Geometry: final body of the model. Coordinates: model frame, mm. A direction names the side the tool comes from. Give positions to 0.01 mm unless a question says otherwise; leave off trailing zeros. Write each loop counter-clockwise with the first axis right and the second up, starting at its lowest first coordinate (ties: lowest second). Pieces come first, ordered by that corner, then holes.
Autodesk Inventor part; units mm, degrees
ref_plane "YZ Plane" through (0, 0, 0) normal (1, 0, 0) x (0, 1, 0)
ref_plane "XZ Plane" through (0, 0, 0) normal (0, 1, 0) x (-1, 0, 0)
ref_plane "XY Plane" through (0, 0, 0) normal (0, 0, 1) x (1, 0, 0)
sketch "Skizze1" plane through (0, 0, 0) normal (0, 0, 1) x (1, 0, 0)
  line L0 (-17.5, 0) -> (17.5, 0)
  line L1 (0, -17.5) -> (0, 17.5)
  circle A0 centre (0, 0) radius 12.5
  dimension "d0" = 25
extrude "Extrusion1" add sketch "Skizze1" along normal blind 3
sketch "Skizze2" plane through (0, 0, 3) normal (0, 0, 1) x (1, 0, 0)
  circle A0 centre (0, 0) radius 10
  dimension "d3" = 20
extrude "Extrusion2" add sketch "Skizze2" along normal blind 5
thread "Gewinde1"
chamfer "Fase1" distance 0.5 angle 45 3 edges at (-10, 0, 8) (-12.5, 0, 3) (-12.5, 0, 0)
sketch "Skizze3" plane through (0, 0, 0) normal (0, 0, -1) x (-1, 0, 0)
  point P0 (0, 0)
  point P1 (0, 0)
hole "Bohrung1" at (0, 0, 0) direction (0, 0, 1) diameter 11.445 depth 32.814
properties part number "VerteilerVerschluss"
Q1. Pin query (flat end, axial travel): P1, Ø9, axis at x = 0, y = 0, coming from the -Z side; P2, Ø7, axis at x = -5.5, y = 0.5, coming from the +Z side; P3, Ø1, axis at y = 6.5, z = 1, coming from the +X side; P4, Ø1, axis at x = -9.5, z = 4, coming from the +Y side. Return the tip coordinate at first contact, or that it passes through.
Filled sheet:
P1: passes through
P2: stops at z = 8
P3: stops at x = 10.97
P4: stops at y = 4.36
Q2. Ray query, line 1 along Y through (x, z) = (0, 4); line 2 along Z through (x, y) = (-9.75, -5.75); line 3 along Y through (x, z) = (-3, 3.5). Return the intervals inside material, ascending.
Filled sheet:
line 1: y = -10 to -5.72, 5.72 to 10
line 2: z = 0 to 3
line 3: y = -9.54 to -4.87, 4.87 to 9.54
Q3. Access query for faces 4 (the flat face through (5.2, 2.8, 0)), 5 (the flat face through (-5, 9, 3)). Directions: +Z, -Z, +X, -X, +Y, -Y. A direction counts if a zero-diameter tool reaches every point of the face in a straight line with its end or side. Return the directions, or none.
Filled sheet:
face 4: -Z, +X, -X, +Y, -Y
face 5: +Z
Q4. Pull-direction query (X, two-part tool) for faces 1 (the flat face through (0, -6, 8)), 2 (the cylindrical face through (-1.719, 5.458, 4.056)), 3 (the cylindrical face through (11.923, -3.755, 1.486)); classes: released by +X, released by -X, zero draft, split by the parting line, or undercut.
Filled sheet:
face 1: zero draft
face 2: undercut
face 3: split by the parting line
Q5. Section A-A on y = 0. Output: boundary loops of the cut face in (x, z), plus the area to 3 significant figures.
Filled sheet:
outline: (-12.5, 0.5) - (-12, 0) - (-5.72, 0) - (-5.72, 8) - (-9.5, 8) - (-10, 7.5) - (-10, 3) - (-12, 3) - (-12.5, 2.5) - close; (5.72, 0) - (12, 0) - (12.5, 0.5) - (12.5, 2.5) - (12, 3) - (10, 3) - (10, 7.5) - (9.5, 8) - (5.72, 8) - close
area: 82.7 mm2
Q6. Section C-C on z = 5.5. Output: boundary loops of the cut face in (x, y) (1 decimal).
Filled sheet:
outline: circle Ø20 at (0, 0); hole circle Ø11.4 at (0, 0)
